Check sheet for the drawn part. Datum: minimum x, y, z corner. Units: mm. A direction names the side the tool comes from. Round coordinates to 2 decimals unless told otherwise and drop trailing zeros. Loops run counter-clockwise (first coordinate to the right, second up) from the corner with the lowest first, then second, coordinate; pieces in that order, holes last.
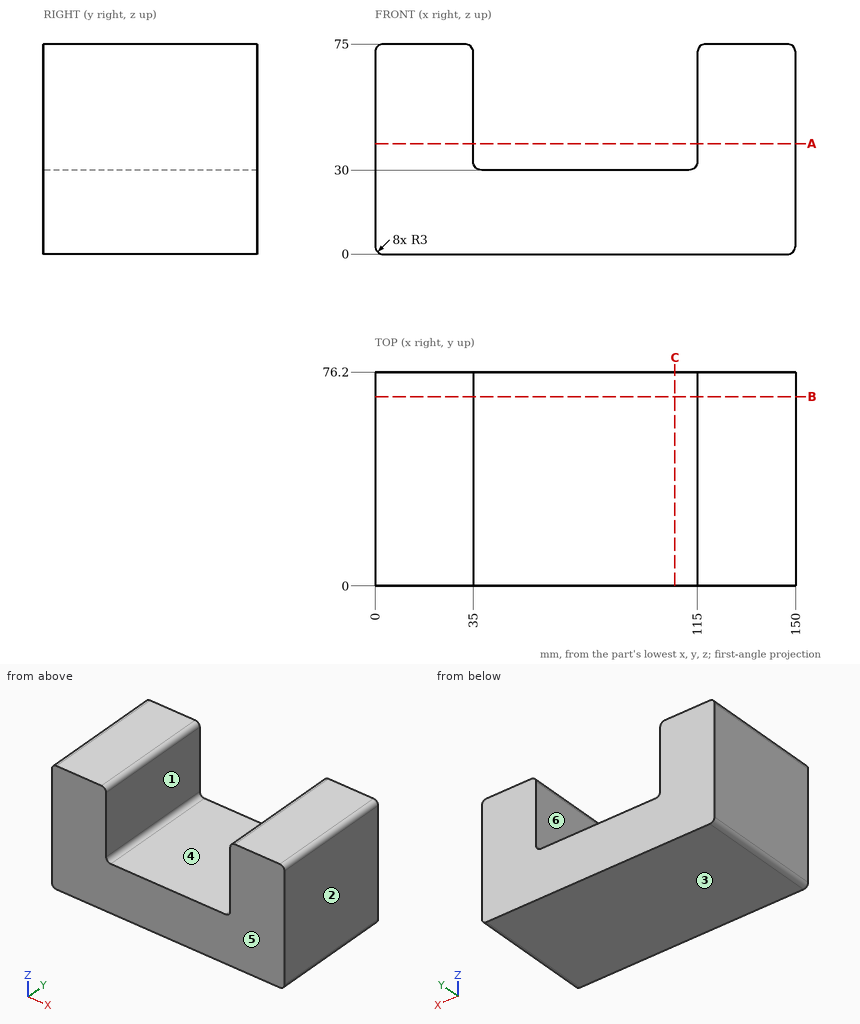
1) Sectioned sample at C-C, the plane x = 107. Record the cut outline in (y, z).
Report:
outline: (0, 0) - (76.2, 0) - (76.2, 30) - (0, 30) - close
2) Mould release check, pull along X, two halves, no side actions. Record for the marked faces 1, 2, 3 and 4: +X half, -X half, draft (parallel to the pull), parting line (faces both ways), or undercut.
Report:
face 1: undercut
face 2: +X half
face 3: draft
face 4: undercut
3) Gauge pin test, flat end, axial feed: pin 1 (10 mm diameter, centred on x = 52.5, y = 7.5, fed in from +Z). Record the tip position at first contact, or that the pin passes through.
Report:
pin 1: stops at z = 30
4) Access from +Z, -Z, +X, -X, +Y, -Y to the whole of each face (thin tool, end or side, straight path). Record for the marked faces 5 and 6.
Report:
face 5: +Z, -Z, +X, -X, -Y
face 6: +Z, +Y, -Y
5) Sectioned sample at B-B, the plane y = 67.5. Record the cut outline in (x, z), then the cut area to 3 significant figures.
Report:
outline: (0, 3) arc R3 ccw to (3, 0) - (147, 0) arc R3 ccw to (150, 3) - (150, 72) arc R3 ccw to (147, 75) - (118, 75) arc R3 ccw to (115, 72) - (115, 33) arc R3 cw to (112, 30) - (38, 30) arc R3 cw to (35, 33) - (35, 72) arc R3 ccw to (32, 75) - (3, 75) arc R3 ccw to (0, 72) - close
area: 7,640 mm2
6) Scan lines: line 1 along X through (y, z) = (36, 58); line 2 along Z through (x, y) = (83, 62); line 3 along Z through (x, y) = (116, 10). Record each from-to range of solid material in increasing order.
Report:
line 1: x = 0 to 35, 115 to 150
line 2: z = 0 to 30
line 3: z = 0 to 74.24
7) Sectioned sample at A-A, the plane z = 39.5. Record the cut outline in (x, y), then the cut area to 3 significant figures.
Report:
outline: (0, 0) - (35, 0) - (35, 76.2) - (0, 76.2) - close; (115, 0) - (150, 0) - (150, 76.2) - (115, 76.2) - close
area: 5,330 mm2
